Design review of the part built by this model. Coordinates are the model's own, in mm. A direction names the side the tool comes from. Give positions to 0.01 mm unless a question says otherwise; leave off trailing zeros. Loops run counter-clockwise (first coordinate to the right, second up) from the corner with the lowest first, then second, coordinate; pieces in that order, holes last. Notation, with made-up numbers: (63, 59.25) -> (73, 59.25) arc R25 cw to (73, 72.25) -> close; hole circle Ø5 at (36, 78). An arc over 180 degrees is marked (long way). Use a Markdown table: item, result. Add a question column.
1. To check wall thickness, follow line 1 (Z direction, x = 25.4, y = 0.55); line 2 (Y direction, x = 146, z = 11.75). State the ranges of each line that lie inside material, in increasing order.
2. For pin 1 Ø1 at (x, z) = (234.5, 2.5) entering from +Y; pin 2 Ø5.5 at (x, y) = (227, 9.5) entering from +Z, all flat-tipped, find the tip position at first contact; note any pin that passes through.
3. Add section A-A (z = 6.7). State the section outline as (x, y) points.
4. Add section C-C (y = 7.75). State the section outline as (x, z) points.
5. Add section B-B (x = 45). State the section outline as (y, z) points.
6. For faces 1 (the flat face through (0, 3, 1)), 2 (the flat face through (188, 7, 1.27)), list the 3-axis set-ups (+Z, -Z, +X, -X, +Y, -Y) from which the entire face can be reached by the end or side of a thin tool; tool diameter is ignored.
```python
from build123d import *

# Parameters (mm, degrees)
F1_DEPTH = 381
F2_R     = 2.5
F3_DEPTH = 25.4


with BuildPart() as f1:
    # F0 (on Right) → F1 (new body)
    with BuildSketch(Plane.YZ):
        Polygon((0, 12.7), (0, 0), (12.7, 0), (12.7, 1.27), (1.27, 1.27), (1.27, 12.7), align=None)
    extrude(amount=F1_DEPTH)

    # F2 (on face) → F3 (cut)
    with BuildSketch(Plane.XZ):
        with Locations((25.4, 6.7)):
            Circle(F2_R)
    extrude(amount=-F3_DEPTH, mode=Mode.SUBTRACT)


solid = f1.part
```
Taken from the geometry:
| question | item | result |
|---|---|---|
| 1 | line 1 | z = 0 to 4.2, 9.2 to 12.7 |
| 1 | line 2 | y = 0 to 1.27 |
| 2 | pin 1 | stops at y = 1.27 |
| 2 | pin 2 | stops at z = 1.27 |
| 3 | outline | (0, 0) -> (22.9, 0) -> (22.9, 1.27) -> (0, 1.27) -> close; (27.9, 0) -> (381, 0) -> (381, 1.27) -> (27.9, 1.27) -> close |
| 4 | outline | (0, 0) -> (381, 0) -> (381, 1.27) -> (0, 1.27) -> close |
| 5 | outline | (0, 0) -> (12.7, 0) -> (12.7, 1.27) -> (1.27, 1.27) -> (1.27, 12.7) -> (0, 12.7) -> close |
| 6 | face 1 | +Z, -Z, -X, +Y, -Y |
| 6 | face 2 | +Z, +X, -X, +Y |
